from build123d import *

# Parameters (mm, degrees)
ESQUISSE1_W             = 80
ESQUISSE1_H             = 12
BOSS_EXTRU_1_DEPTH      = 9
ESQUISSE2_W             = 10
ESQUISSE2_H             = 9
BOSS_EXTRU_2_DEPTH      = 9
ESQUISSE3_R             = 2.1
ENL_V_MAT_EXTRU_1_DEPTH = 84.19855768


with BuildPart() as part:
    # Esquisse1 → Boss.-Extru.1 (new body)
    with BuildSketch(Plane.XY):
        with Locations((40, 6)):
            Rectangle(ESQUISSE1_W, ESQUISSE1_H)
    extrude(amount=BOSS_EXTRU_1_DEPTH)

    # Esquisse2 → Boss.-Extru.2 (add)
    with BuildSketch(Plane.XY.offset(9)):
        with Locations((5, 16.5)):
            Rectangle(ESQUISSE2_W, ESQUISSE2_H)
        with Locations((25, 16.5)):
            Rectangle(ESQUISSE2_W, ESQUISSE2_H)
    extrude(amount=-BOSS_EXTRU_2_DEPTH)

    # Esquisse3 → Enlèv. mat.-Extru.1 (cut, through all)
    with BuildSketch(Plane.XY.offset(9)):
        with Locations((63, 6)):
            Circle(ESQUISSE3_R)
        with Locations((75, 6)):
            Circle(ESQUISSE3_R)
    extrude(amount=-ENL_V_MAT_EXTRU_1_DEPTH, mode=Mode.SUBTRACT)


solid = part.part
Work out the finished part from the listing and answer in its coordinate system (mm). A direction names the side the tool comes from. Give positions to 0.01 mm unless a question says otherwise; leave off trailing zeros. Order: outer loops, then holes, each group sorted by start corner. A loop starts at its lowest first (then second) coordinate and runs counter-clockwise, first axis right, second up. Notation, with made-up numbers: (67, 79) - (123, 79) arc R11 cw to (123, 93) - close; hole circle Ø5 at (37.5, -38). An arc over 180 degrees is marked (long way). Answer as CSV lines item,"result". Start each with the question number.
Q1. Find the intervals of material crossed by L1, parallel to Y at x = 75, z = 4.25; L2, parallel to X at y = 14.5, z = 4.75; L3, parallel to X at y = 4.25, z = 0.5, in increasing order. Write a range as [from, to].
Q2. The part is cut by section C-C (x = 75). Write down the section's boundary in (y, z), then the cut area to 3 significant figures.
Q3. The part is cut by section A-A (y = 6). Write down the section's boundary in (x, z), then the cut area to 3 significant figures.
Q4. For faces 4 (the face through (55, 12, 4)), 5 (the face through (20, 16, 5)), 6 (the face through (72.9, 6.09, 4.56)), determine the directions among +Z, -Z, +X, -X, +Y, -Y from which every point of the face is accessible in a straight line to the end or side of a thin tool.
Q5. The part is cut by section B-B (z = 5.5). Write down the section's boundary in (x, y), then the cut area to 3 significant figures.
Q6. The mould has two halves that part along X. Classify faces 1 (the face through (5, 21, 5)), 2 (the face through (30, 16, 5)), 3 (the face through (15, 12, 4)): +X half, -X half, draft (parallel to the pull), parting line (faces both ways), or undercut.
Q7. The part is cut by section D-D (y = 17). Write down the section's boundary in (x, z), then the cut area to 3 significant figures.
Q8. Given pin 1 Ø1.5 at (x, z) = (56, 3.5) entering from +Y; pin 2 Ø2.5 at (x, y) = (63, 6) entering from -Z; pin 3 Ø1.5 at (y, z) = (16, 3) entering from +X, each flat-ended and moving along its own axis, determine where each tip first touches the part or whether it passes through.
Check result:
1,L1,"y = [0, 3.9], [8.1, 12]"
1,L2,"x = [0, 10], [20, 30]"
1,L3,"x = [0, 61.84], [64.16, 73.84], [76.16, 80]"
2,outline,"(0, 0) - (3.9, 0) - (3.9, 9) - (0, 9) - close; (8.1, 0) - (12, 0) - (12, 9) - (8.1, 9) - close"
2,area,"70.2 mm²"
3,outline,"(0, 0) - (60.9, 0) - (60.9, 9) - (0, 9) - close; (65.1, 0) - (72.9, 0) - (72.9, 9) - (65.1, 9) - close; (77.1, 0) - (80, 0) - (80, 9) - (77.1, 9) - close"
3,area,"644 mm²"
4,face 4,"+Z, -Z, +X, +Y"
4,face 5,"+Z, -Z, +Y"
4,face 6,"+Z, -Z"
5,outline,"(0, 0) - (80, 0) - (80, 12) - (30, 12) - (30, 21) - (20, 21) - (20, 12) - (10, 12) - (10, 21) - (0, 21) - close; hole circle Ø4.2 at (63, 6); hole circle Ø4.2 at (75, 6)"
5,area,"1,110 mm²"
6,face 1,"draft"
6,face 2,"+X half"
6,face 3,"undercut"
7,outline,"(0, 0) - (10, 0) - (10, 9) - (0, 9) - close; (20, 0) - (30, 0) - (30, 9) - (20, 9) - close"
7,area,"180 mm²"
8,pin 1,"stops at y = 12"
8,pin 2,"passes through"
8,pin 3,"stops at x = 30"
